```python
from build123d import *

# Parameters (mm, degrees)
SKETCH1_W           = 17
SKETCH1_H           = 17
BOSS_EXTRUDE1_DEPTH = 625
CUT_EXTRUDE1_DEPTH  = 626.639672655
CUT_EXTRUDE9_DEPTH  = 3


with BuildPart() as part:
    # Sketch1 → Boss-Extrude1 (new body)
    with BuildSketch(Plane(origin=(0, 0, 0), x_dir=(1, 0, 0), z_dir=(0, 1, 0))):
        with BuildLine():
            Line((0.5, 0), (19.5, 0))
            ThreePointArc((19.5, 0), (19.853553391, 0.146446609), (20, 0.5))
            Line((20, 0.5), (20, 19.5))
            ThreePointArc((20, 19.5), (19.853553391, 19.853553391), (19.5, 20))
            Line((19.5, 20), (0.5, 20))
            ThreePointArc((0.5, 20), (0.146446609, 19.853553391), (0, 19.5))
            Line((0, 19.5), (0, 0.5))
            ThreePointArc((0, 0.5), (0.146446609, 0.146446609), (0.5, 0))
        make_face()
        with Locations((10, 10)):
            Rectangle(SKETCH1_W, SKETCH1_H, mode=Mode.SUBTRACT)
    extrude(amount=BOSS_EXTRUDE1_DEPTH)

    # Sketch2 → Cut-Extrude1 (cut, through all)
    with BuildSketch(Plane.XY):
        Polygon((9.404700538, 15.155444566), (3, 26.248711306), (3, 34.641016151), (0, 34.641016151), (0, 0), (20, 0), (20, 2), (17, 2), (14.404700538, 6.495190528), (7.476497308, 2.495190528), (2.476497308, 11.155444566), align=None)
    extrude(amount=-CUT_EXTRUDE1_DEPTH, mode=Mode.SUBTRACT)

    # Sketch4 → Cut-Extrude9 (cut)
    with BuildSketch(Plane.XY):
        Polygon((20, 595), (20, 560.358983849), (17, 560.358983849), (17, 565.555136271), (3, 589.803847577), (0, 589.803847577), (0, 595), align=None)
    cut_extrude9 = extrude(amount=-CUT_EXTRUDE9_DEPTH, mode=Mode.SUBTRACT)

    # Mirror2: Cut-Extrude9 across plane
    add(cut_extrude9.mirror(Plane.XY.offset(-10)), mode=Mode.SUBTRACT)


solid = part.part
```
Part model, mm, in its own coordinate system. A direction names the side the tool comes from. Round coordinates to 2 decimals unless told otherwise and drop trailing zeros. Loops run counter-clockwise (first coordinate to the right, second up) from the corner with the lowest first, then second, coordinate; pieces in that order, holes last.
Item 1: Mould opens along X. For faces 4 (the face through (10, 610, -1.5)), 5 (the face through (20, 309, -10)), 6 (the face through (10, 292, -20)) say: +X half, -X half, draft (parallel to the pull), parting line (faces both ways), or undercut.
Item 2: 3-axis set-ups, long thin cutter, end or side, ignore diameter. For faces 1 (the face through (10.1, 577.51, -0.74)), 2 (the face through (1.5, 326, -10)), 3 (the face through (10, 292, 0)): which of +Z, -Z, +X, -X, +Y, -Y reach the whole face in a straight line?
Item 3: Drop flat-ended pins along their axis: P1, Ø0.9, axis at x = 2, z = -9.5, coming from the -Y side; P2, Ø0.9, axis at x = 6.5, z = -18.5, coming from the -Y side; P3, Ø1.5, axis at x = 14.5, z = -2, coming from the -Y side; P4, Ø1.2, axis at x = 19, y = 579, coming from the +Z side. Give the stop position or say it passes through.
Item 4: Drill centre lines: line 1 (Z direction, x = 17.75, y = 63.5); line 2 (Y direction, x = 5.25, z = -1.25); line 3 (X direction, y = 240, z = -16.75). Where is each one in solid material? Low to high.
Item 5: Cut at B-B, the plane y = 315. Give the cut face in (x, z).
Item 6: Cut at A-A, the plane z = -6.75. Give the cut face in (x, y).
A:
1. face 4: undercut
1. face 5: +X half
1. face 6: draft
2. face 1: +Z, -Z, +X
2. face 2: +Y, -Y
2. face 3: +Z, +X, -X, +Y, -Y
3. P1: passes through
3. P2: stops at y = 3.41
3. P3: stops at y = 5.36
3. P4: stops at z = -3
4. line 1: z = -20 to -18.5, -1.5 to 0
4. line 2: y = 6.35 to 12.76, 22.35 to 585.91, 595 to 625
4. line 3: x = 0 to 1.5, 18.5 to 20
5. outline: (0, -19.5) arc R0.5 ccw to (0.5, -20) - (19.5, -20) arc R0.5 ccw to (20, -19.5) - (20, -0.5) arc R0.5 ccw to (19.5, 0) - (0.5, 0) arc R0.5 ccw to (0, -0.5) - close; hole (1.5, -18.5) - (18.5, -18.5) - (18.5, -1.5) - (1.5, -1.5) - close
6. outline: (0, 34.64) - (1.5, 34.64) - (1.5, 625) - (0, 625) - close; (18.5, 2) - (20, 2) - (20, 625) - (18.5, 625) - close
